Can you work these out from the model? Positions are in its coordinate system, mm. A direction names the side the tool comes from. Round coordinates to 2 decimals unless told otherwise and drop trailing zeros. Loops run counter-clockwise (first coordinate to the right, second up) from the corner with the lowest first, then second, coordinate; pieces in that order, holes last. Notation, with made-up numbers: (1, 18.25) -> (47, 18.25) arc R36 cw to (47, 53.25) -> close; hole circle Ø9 at (3, 28). An arc over 180 degrees is marked (long way). Write each question's results on one line, items separated by ' | '.
from build123d import *

# Parameters (mm, degrees)
BOSS_EXTRUDE1_DEPTH            = 27.5
CUT_EXTRUDE2_START             = 27.5
CUT_EXTRUDE2_DEPTH             = 25
CUT_EXTRUDE3_START             = -2
SKETCH3_R                      = 8.5
CUT_EXTRUDE3_DEPTH             = 6
CUT_EXTRUDE4_START             = -9
SKETCH4_R                      = 8.5
CUT_EXTRUDE4_DEPTH             = 6
CUT_EXTRUDE6_DEPTH             = 72.98958258
M3_CLEARANCE_HOLE1_D           = 3.6
M3_CLEARANCE_HOLE1_DEPTH       = 26.4
M3_CLEARANCE_HOLE1_TIP         = 1.081549114
SKETCH16_W                     = 4
SKETCH16_H                     = 27.5
CUT_EXTRUDE7_DEPTH             = 10
CUT_EXTRUDE8_START             = -2
SKETCH17_R                     = 8.5
CUT_EXTRUDE8_DEPTH             = 6
CUT_EXTRUDE9_REACH             = 98.152
CHAMFER1_SIZE                  = 2
CHAMFER1_SIZE2                 = 4.289013841
CHAMFER2_SIZE                  = 6
CHAMFER2_SIZE_2                = 12.867041523
CUT_EXTRUDE10_DEPTH            = 64.863134906
CUT_EXTRUDE10_DEPTH_BACK       = 64.863134906
SKETCH18_W                     = 3
SKETCH18_H                     = 7
SKETCH19_W                     = 32
SKETCH19_H                     = 4
CUT_EXTRUDE12_DEPTH            = 10
CUT_EXTRUDE13_START            = -83
SKETCH19_2_W                   = 32
SKETCH19_2_H                   = 4
CUT_EXTRUDE13_DEPTH            = 10
F_5_3_5_3_DIAMETER_HOLE1_D     = 5.3
F_5_3_5_3_DIAMETER_HOLE1_DEPTH = 5
F_5_3_5_3_DIAMETER_HOLE1_TIP   = 1.59228064
F_5_3_5_3_DIAMETER_HOLE2_D     = 5.3
F_5_3_5_3_DIAMETER_HOLE2_DEPTH = 5
F_5_3_5_3_DIAMETER_HOLE2_TIP   = 1.59228064
M3_CLEARANCE_HOLE2_D           = 3.6
M3_CLEARANCE_HOLE2_DEPTH       = 26.4
M3_CLEARANCE_HOLE2_TIP         = 1.081549114
CHAMFER3_SIZE                  = 2
CHAMFER4_SIZE                  = 2
CHAMFER5_SIZE                  = 2


with BuildPart() as part:
    # Sketch1 → Boss-Extrude1 (new body)
    with BuildSketch(Plane(origin=(0, 0, 0), x_dir=(1, 0, 0), z_dir=(0, 1, 0))):
        Polygon((-41.5, 12), (41.5, 12), (41.5, -30), (23, -30), (23, -40), (-23, -40), (-23, -30), (-41.5, -30), align=None)
    extrude(amount=BOSS_EXTRUDE1_DEPTH)

    # Sketch1<4> → Cut-Extrude2 (cut)
    with BuildSketch(Plane(origin=(0, 0, 0), x_dir=(1, 0, 0), z_dir=(0, 1, 0)).offset(CUT_EXTRUDE2_START)):
        Polygon((31.5, 0), (-31.5, 0), (-31.5, -25), (-18, -25), (-18, -30), (18, -30), (18, -25), (31.5, -25), (31.5, -10), align=None)
    extrude(amount=-CUT_EXTRUDE2_DEPTH, mode=Mode.SUBTRACT)

    # Sketch3 → Cut-Extrude3 (cut)
    with BuildSketch(Plane.XY.offset(40).offset(CUT_EXTRUDE3_START)):
        with Locations((0, 27.5)):
            Circle(SKETCH3_R)
    extrude(amount=-CUT_EXTRUDE3_DEPTH, mode=Mode.SUBTRACT)

    # Sketch4 → Cut-Extrude4 (cut)
    with BuildSketch(Plane(origin=(0, 0, -12), x_dir=(-1, 0, 0), z_dir=(0, 0, -1)).offset(CUT_EXTRUDE4_START)):
        with Locations((0, 27.5)):
            Circle(SKETCH4_R)
    extrude(amount=CUT_EXTRUDE4_DEPTH, mode=Mode.SUBTRACT)

    # Sketch3<4> → Cut-Extrude6 (cut, through all)
    with BuildSketch(Plane.XY.offset(40)):
        with BuildLine():
            Line((-7, 27.5), (7, 27.5))
            ThreePointArc((7, 27.5), (0, 34.5), (-7, 27.5))
        make_face()
        with BuildLine():
            ThreePointArc((-7, 27.5), (0, 20.5), (7, 27.5))
            Line((7, 27.5), (-7, 27.5))
        make_face()
        with BuildLine():
            Line((-7, 27.5), (7, 27.5))
            ThreePointArc((7, 27.5), (0, 34.5), (-7, 27.5))
        make_face()
        with BuildLine():
            ThreePointArc((-7, 27.5), (0, 20.5), (7, 27.5))
            Line((7, 27.5), (-7, 27.5))
        make_face()
    extrude(amount=-CUT_EXTRUDE6_DEPTH, mode=Mode.SUBTRACT)

    # M3 Clearance Hole1
    with Locations(Plane(origin=(41.5, 0, 0), x_dir=(0, 0, -1), z_dir=(1, 0, 0))):
        with Locations((8.5, 4), (-36.5, 4), (8.5, 24), (-36.5, 24)):
            Hole(M3_CLEARANCE_HOLE1_D / 2, depth=M3_CLEARANCE_HOLE1_DEPTH)
            with Locations((0, 0, -(M3_CLEARANCE_HOLE1_DEPTH + M3_CLEARANCE_HOLE1_TIP / 2))):  # 118° drill point
                Cone(0, M3_CLEARANCE_HOLE1_D / 2, M3_CLEARANCE_HOLE1_TIP, mode=Mode.SUBTRACT)

    # Sketch16 → Cut-Extrude7 (cut)
    with BuildSketch(Plane(origin=(0, 0, -12), x_dir=(-1, 0, 0), z_dir=(0, 0, -1))):
        with Locations((25, 13.75)):
            Rectangle(SKETCH16_W, SKETCH16_H)
        with Locations((-25, 13.75)):
            Rectangle(SKETCH16_W, SKETCH16_H)
    extrude(amount=-CUT_EXTRUDE7_DEPTH, mode=Mode.SUBTRACT)

    # Sketch17 → Cut-Extrude8 (cut)
    with BuildSketch(Plane(origin=(41.5, 0, 0), x_dir=(0, 0, -1), z_dir=(1, 0, 0)).offset(CUT_EXTRUDE8_START)):
        with Locations((-14, 27.5)):
            Circle(SKETCH17_R)
    extrude(amount=-CUT_EXTRUDE8_DEPTH, mode=Mode.SUBTRACT)

    # Cut-Extrude9: up to this face of the body (flat: up to its plane)
    cut_extrude9_end = Plane(part.part.faces().sort_by_distance((31.5, 15, 12.5))[0])
    # Sketch17<3> → Cut-Extrude9 (cut, up to the picked face)
    with BuildSketch(Plane(origin=(41.5, 0, 0), x_dir=(0, 0, -1), z_dir=(1, 0, 0)), mode=Mode.PRIVATE) as cut_extrude9_sk1:
        with BuildLine():
            Line((-21, 27.5), (-7, 27.5))
            ThreePointArc((-7, 27.5), (-14, 34.5), (-21, 27.5))
        make_face()
    cut_extrude9_tool1 = split(extrude(cut_extrude9_sk1.sketch, amount=-CUT_EXTRUDE9_REACH, mode=Mode.PRIVATE), bisect_by=cut_extrude9_end, keep=Keep.BOTH, mode=Mode.PRIVATE)
    # Sketch17<3> → Cut-Extrude9 (cut, up to the picked face)
    with BuildSketch(Plane(origin=(41.5, 0, 0), x_dir=(0, 0, -1), z_dir=(1, 0, 0)), mode=Mode.PRIVATE) as cut_extrude9_sk2:
        with BuildLine():
            ThreePointArc((-21, 27.5), (-14, 20.5), (-7, 27.5))
            Line((-7, 27.5), (-21, 27.5))
        make_face()
    cut_extrude9_tool2 = split(extrude(cut_extrude9_sk2.sketch, amount=-CUT_EXTRUDE9_REACH, mode=Mode.PRIVATE), bisect_by=cut_extrude9_end, keep=Keep.BOTH, mode=Mode.PRIVATE)
    # Sketch17<3> → Cut-Extrude9 (cut, up to the picked face)
    with BuildSketch(Plane(origin=(41.5, 0, 0), x_dir=(0, 0, -1), z_dir=(1, 0, 0)), mode=Mode.PRIVATE) as cut_extrude9_sk3:
        with BuildLine():
            Line((-21, 27.5), (-7, 27.5))
            ThreePointArc((-7, 27.5), (-14, 34.5), (-21, 27.5))
        make_face()
    cut_extrude9_tool3 = split(extrude(cut_extrude9_sk3.sketch, amount=-CUT_EXTRUDE9_REACH, mode=Mode.PRIVATE), bisect_by=cut_extrude9_end, keep=Keep.BOTH, mode=Mode.PRIVATE)
    # Sketch17<3> → Cut-Extrude9 (cut, up to the picked face)
    with BuildSketch(Plane(origin=(41.5, 0, 0), x_dir=(0, 0, -1), z_dir=(1, 0, 0)), mode=Mode.PRIVATE) as cut_extrude9_sk4:
        with BuildLine():
            ThreePointArc((-21, 27.5), (-14, 20.5), (-7, 27.5))
            Line((-7, 27.5), (-21, 27.5))
        make_face()
    cut_extrude9_tool4 = split(extrude(cut_extrude9_sk4.sketch, amount=-CUT_EXTRUDE9_REACH, mode=Mode.PRIVATE), bisect_by=cut_extrude9_end, keep=Keep.BOTH, mode=Mode.PRIVATE)
    add(cut_extrude9_tool1.solids().sort_by(Axis((41.5, 30.470892, 14), (-1, 0, 0)))[0], mode=Mode.SUBTRACT)
    add(cut_extrude9_tool2.solids().sort_by(Axis((41.5, 24.529108, 14), (-1, 0, 0)))[0], mode=Mode.SUBTRACT)
    add(cut_extrude9_tool3.solids().sort_by(Axis((41.5, 30.470892, 14), (-1, 0, 0)))[0], mode=Mode.SUBTRACT)
    add(cut_extrude9_tool4.solids().sort_by(Axis((41.5, 24.529108, 14), (-1, 0, 0)))[0], mode=Mode.SUBTRACT)

    # Chamfer1
    chamfer1_edges = [part.edges().sort_by_distance(p)[0] for p in [
        (23, 13.75, 30),
    ]]
    chamfer1_side = [part.faces().sort_by_distance(p)[0] for p in [
        (23, 13.730013625, 34.88008175),
    ]]
    chamfer(chamfer1_edges, length=CHAMFER1_SIZE, length2=CHAMFER1_SIZE2, reference=chamfer1_side[0])

    # Chamfer2
    # the kernel refuses this chamfer: 12.867041523, 6 mm, written as the material it takes off along each edge
    with BuildSketch(Plane(origin=(18, 60.838188976, 25), x_dir=(-0.07481330637059953, 0, 0.9971975577536775), z_dir=(0, -1, 0))) as chamfer2_piece_1_section:
        Polygon((CHAMFER2_SIZE * 0.997197557754, -CHAMFER2_SIZE * 0.0748133063706), (-CHAMFER2_SIZE_2 * 0.0748133063709, -CHAMFER2_SIZE_2 * 0.997197557758), (0, 0), align=None)
    chamfer2_piece_1 = extrude(amount=58.338188976, mode=Mode.PRIVATE)
    chamfer2_piece_1 = split(chamfer2_piece_1, bisect_by=Plane(origin=(22.391133218, 15, 30), z_dir=(0, 0, -1)), keep=Keep.TOP, mode=Mode.PRIVATE)
    add(chamfer2_piece_1, mode=Mode.SUBTRACT)

    # Sketch18 → Cut-Extrude10 (cut, two sides: drawn at the far end of the back side and taken through both)
    with BuildSketch(Plane(origin=(0, 27.5, 0), x_dir=(1, 0, 0), z_dir=(0, 1, 0)).offset(-CUT_EXTRUDE10_DEPTH_BACK)):
        with Locations((-15.5, 8.5)):
            Rectangle(SKETCH18_W, SKETCH18_H)
        with Locations((15.5, 8.5)):
            Rectangle(SKETCH18_W, SKETCH18_H)
        with Locations((-15.5, -36.5)):
            Rectangle(SKETCH18_W, SKETCH18_H)
        with Locations((15.5, -36.5)):
            Rectangle(SKETCH18_W, SKETCH18_H)
    extrude(amount=CUT_EXTRUDE10_DEPTH + CUT_EXTRUDE10_DEPTH_BACK, mode=Mode.SUBTRACT)

    # Sketch19 → Cut-Extrude12 (cut)
    with BuildSketch(Plane.ZY.offset(41.5)):
        with Locations((14, 2)):
            Rectangle(SKETCH19_W, SKETCH19_H)
    extrude(amount=-CUT_EXTRUDE12_DEPTH, mode=Mode.SUBTRACT)

    # Sketch19<2> → Cut-Extrude13 (cut)
    with BuildSketch(Plane.ZY.offset(41.5).offset(CUT_EXTRUDE13_START)):
        with Locations((14, 2)):
            Rectangle(SKETCH19_2_W, SKETCH19_2_H)
    extrude(amount=CUT_EXTRUDE13_DEPTH, mode=Mode.SUBTRACT)

    # Ø5.3 (5.3) Diameter Hole1
    with Locations(Plane(origin=(0, 4, 0), x_dir=(-1, 0, 0), z_dir=(0, -1, 0))):
        with Locations((36.5, -24), (36.5, -4), (-36.5, -24), (-36.5, -4)):
            Hole(F_5_3_5_3_DIAMETER_HOLE1_D / 2, depth=F_5_3_5_3_DIAMETER_HOLE1_DEPTH)
            with Locations((0, 0, -(F_5_3_5_3_DIAMETER_HOLE1_DEPTH + F_5_3_5_3_DIAMETER_HOLE1_TIP / 2))):  # 118° drill point
                Cone(0, F_5_3_5_3_DIAMETER_HOLE1_D / 2, F_5_3_5_3_DIAMETER_HOLE1_TIP, mode=Mode.SUBTRACT)

    # Ø5.3 (5.3) Diameter Hole2
    with Locations(Plane(origin=(0, 27.5, 0), x_dir=(1, 0, 0), z_dir=(0, 1, 0))):
        with Locations((-36.5, 0), (-36.5, -20), (36.5, 0)):
            Hole(F_5_3_5_3_DIAMETER_HOLE2_D / 2, depth=F_5_3_5_3_DIAMETER_HOLE2_DEPTH)
            with Locations((0, 0, -(F_5_3_5_3_DIAMETER_HOLE2_DEPTH + F_5_3_5_3_DIAMETER_HOLE2_TIP / 2))):  # 118° drill point
                Cone(0, F_5_3_5_3_DIAMETER_HOLE2_D / 2, F_5_3_5_3_DIAMETER_HOLE2_TIP, mode=Mode.SUBTRACT)

    # M3 Clearance Hole2
    with Locations(Plane.ZY.offset(41.5)):
        with Locations((-8.5, 24), (36.5, 24), (36.5, 4), (-8.5, 4)):
            Hole(M3_CLEARANCE_HOLE2_D / 2, depth=M3_CLEARANCE_HOLE2_DEPTH)
            with Locations((0, 0, -(M3_CLEARANCE_HOLE2_DEPTH + M3_CLEARANCE_HOLE2_TIP / 2))):  # 118° drill point
                Cone(0, M3_CLEARANCE_HOLE2_D / 2, M3_CLEARANCE_HOLE2_TIP, mode=Mode.SUBTRACT)

    # Chamfer3
    # the kernel refuses this chamfer: 2 mm, written as the material it adds along each edge
    with BuildSketch(Plane(origin=(25.287872896, 2.5, 30), x_dir=(0, -0.027495876610586296, -0.9996219169112968), z_dir=(-1, 0, 0))) as chamfer3_piece_1:
        Polygon((CHAMFER3_SIZE * 0.999621916911, -CHAMFER3_SIZE * 0.0274958766106), (-CHAMFER3_SIZE * 0.0274958766106, -CHAMFER3_SIZE * 0.999621916911), (0, 0), align=None)
    extrude(amount=48.431238872)
    with BuildSketch(Plane(origin=(31.5, 2.5, 0), x_dir=(0, -0.027495876610586275, 0.9996219169112968), z_dir=(-1, 0, 0))) as chamfer3_piece_2:
        Polygon((CHAMFER3_SIZE * 0.999621916911, CHAMFER3_SIZE * 0.0274958766106), (-CHAMFER3_SIZE * 0.0274958766106, CHAMFER3_SIZE * 0.999621916911), (0, 0), align=None)
    extrude(amount=63)
    # the kernel refuses this chamfer: 2 mm, written as the material it takes off along each edge
    with BuildSketch(Plane(origin=(27, 0, -2), x_dir=(0, -0.027495876610586355, 0.9996219169112968), z_dir=(-1, 0, 0)), Plane(origin=(-23, 0, -2), x_dir=(0, -0.027495876610586382, 0.9996219169112968), z_dir=(-1, 0, 0))) as chamfer3_2_piece_1:
        Polygon((CHAMFER3_SIZE * 0.999621916911, CHAMFER3_SIZE * 0.0274958766106), (-CHAMFER3_SIZE * 0.0274958766106, CHAMFER3_SIZE * 0.999621916911), (0, 0), align=None)
    extrude(amount=4, mode=Mode.SUBTRACT)
    with BuildSketch(Plane(origin=(-23, 0, 30), x_dir=(0, -0.02749587661058639, -0.9996219169112968), z_dir=(-1, 0, 0))) as chamfer3_2_piece_2:
        Polygon((CHAMFER3_SIZE * 0.999621916911, -CHAMFER3_SIZE * 0.0274958766106), (-CHAMFER3_SIZE * 0.0274958766106, -CHAMFER3_SIZE * 0.999621916911), (0, 0), align=None)
    extrude(amount=13.643365976, mode=Mode.SUBTRACT)

    # Chamfer4
    chamfer4_edges = [part.edges().sort_by_distance(p)[0] for p in [
        (27.650281142, 2.5, 26.5),
    ]]
    chamfer(chamfer4_edges, length=CHAMFER4_SIZE)

    # Chamfer5
    chamfer5_edges = [part.edges().sort_by_distance(p)[0] for p in [
        (29.394506921, 0, 30),
        (25.144506921, 0, 31),
    ]]
    chamfer(chamfer5_edges, length=CHAMFER5_SIZE)


solid = part.part
1. Please list where these lines run through material, in increasing order: line 1 (X direction, y = 7.75, z = -7); line 2 (X direction, y = 24.25, z = 20); line 3 (Z direction, x = -36.5, y = 6). Write a range as from..to.
Final values:
line 1: -41.5..-27, -23..-17, -14..14, 17..23, 27..41.5 | line 2: -41.5..-39.15, -33.85..-31.5 | line 3: -12..1.35, 6.65..21.35, 26.65..30
2. On a 3-axis mill with a long thin cutter (end or side, diameter ignored), from which of +Z, -Z, +X, -X, +Y, -Y can I reach the whole of each face in a straight line? I mean faces 4 (the face through (-25, 1, -1)), 5 (the face through (-19.96, 4.08, -6.7)), 6 (the face through (37, 2, -2)), 7 (the face through (32.51, 20.5, 14.15)), 8 (the face through (0, 20, 38)). Say none if no direction works.
Final values:
face 4: -Z, -Y | face 5: -X | face 6: +Z, +X, -Y | face 7: +X, +Y | face 8: +Y
3. If we section it at C-C (z = 14): List the corners of the cut face in (x, y) for me, then the cut area to 4 significant figures.
Final values:
outline: (-41.5, 4) -> (-31.5, 4) -> (-31.5, 27.5) -> (-41.5, 27.5) -> close; (-31.5, 0) -> (31.5, 0) -> (31.5, 2.5) -> (-31.5, 2.5) -> close; (31.5, 4) -> (41.5, 4) -> (41.5, 20.5) -> (39.5, 20.5) -> (39.5, 19) -> (33.5, 19) -> (33.5, 20.5) -> (31.5, 20.5) -> close | area: 548.5 mm2
4. If we section it at B-B (x = 0): List the corners of the cut face in (y, z) for me, then the cut area to 3 significant figures.
Final values:
outline: (0, -12) -> (20.5, -12) -> (20.5, -9) -> (19, -9) -> (19, -3) -> (20.5, -3) -> (20.5, 0) -> (4.5, 0) -> (2.5, 2) -> (2.5, 28) -> (4.5, 30) -> (20.5, 30) -> (20.5, 32) -> (19, 32) -> (19, 38) -> (20.5, 38) -> (20.5, 40) -> (0, 40) -> close | area: 512 mm2
5. Will these pins go through, and if not, where does the flat tip stop? pin 1 (1 mm diameter, centred on x = -29, y = 19.5, fed in from +Z); pin 2 (2 mm diameter, centred on y = 8.5, z = 35, fed in from +X); pin 3 (5 mm diameter, centred on x = 7, z = 11, fed in from +Y).
Final values:
pin 1: z = 30 | pin 2: x = 23 | pin 3: y = 2.5
6. If we section it at A-A (z = 36.5): State how many separate pieces and enclosed holes the cut face has, then the cut area to 3 significant figures.
Final values:
separate pieces: 7 | enclosed holes: 0 | area: 900 mm2
7. We'd pull the mould along Y, two halves only. Please class faces 1 (the face through (-37, 4, 14)), 2 (the face through (0, 16, 0)), 3 (the face through (34.15, 4.08, -10.3)): pulls with the +Y half, pulls with the -Y half, needs draft (parallel to the pull), parting line crosses it, or undercut.
Final values:
face 1: pulls with the -Y half | face 2: needs draft | face 3: undercut
